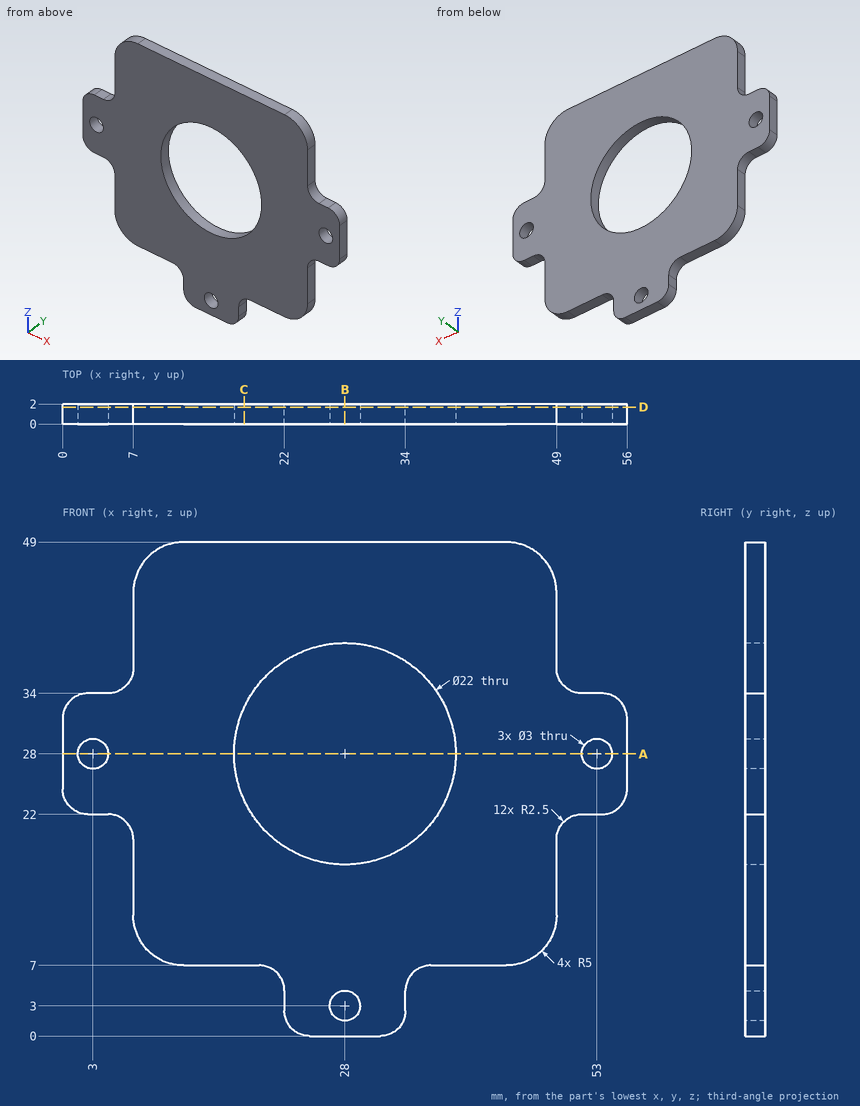
Part print with two shaded views. Sizes in mm from the minimum x, y, z corner. Coordinates: 2 decimals unless noted, no trailing zeros. Order: outer loops, then holes, each group sorted by start corner. A loop starts at its lowest first (then second) coordinate and runs counter-clockwise, first axis right, second up. Notation, with made-up numbers: M -24,-32.75 L 30,-32.75 A12 cw 30,-10.75 Z; hole C -24,-13.75 d6. An arc over 180 degrees is marked long. One line per question, with ' | ' between items. Start each with the question number.
1. Cut at C-C (x = 18). Write the cut outline in (y, z).
2. Cut at B-B (x = 28). Write the cut outline in (y, z).
3. Cut at A-A (z = 28). Write the cut outline in (x, y), plus the area to 3 significant figures.
4. Wall check: line 1 along X through (y, z) = (1.15, 28); line 2 along X through (y, z) = (1, 27.5); line 3 along X through (y, z) = (1, 3). Give the ranges that are in metal, low to high. Write a range as [from, to].
5. Cut at D-D (y = 1.7). Count the separate pieces of the cut face and the enclosed holes in it, plus the area to 3 significant figures.
6. Flat gauge pins, fed straight in: P1, Ø0.6, axis at y = 1.5, z = 14.5, coming from the +X side; P2, Ø1, axis at x = 52.5, y = 1, coming from the -Z side; P3, Ø1, axis at y = 1, z = 3, coming from the +X side; P4, Ø8, axis at x = 34.5, z = 24.5, coming from the -Y side. Where does each tip first touch, or does it go through?
The answers:
1) outline: M 0,7 L 2,7 L 2,23.42 L 0,23.42 Z; M 0,32.58 L 2,32.58 L 2,49 L 0,49 Z
2) outline: M 0,0 L 2,0 L 2,1.5 L 0,1.5 Z; M 0,4.5 L 2,4.5 L 2,17 L 0,17 Z; M 0,39 L 2,39 L 2,49 L 0,49 Z
3) outline: M 0,0 L 1.5,0 L 1.5,2 L 0,2 Z; M 4.5,0 L 17,0 L 17,2 L 4.5,2 Z; M 39,0 L 51.5,0 L 51.5,2 L 39,2 Z; M 54.5,0 L 56,0 L 56,2 L 54.5,2 Z | area: 56.0 mm2
4) line 1: x = [0, 1.5], [4.5, 17], [39, 51.5], [54.5, 56] | line 2: x = [0, 1.59], [4.41, 17.01], [38.99, 51.59], [54.41, 56] | line 3: x = [22, 26.5], [29.5, 34]
5) separate pieces: 1 | enclosed holes: 4 | area: 1,590 mm2
6) P1: stops at x = 49 | P2: stops at z = 22 | P3: stops at x = 34 | P4: stops at y = 0
